Autodesk Fusion 360 part; units mm, degrees
sketch "スケッチ1" plane through (0, 0, 0) normal (0, 0, 1) x (1, 0, 0)
  line L0 (0, 0) -> (74, 0)
  line L1 (74, 0) -> (74, 46)
  line L2 (74, 46) -> (0, 46)
  line L3 (0, 46) -> (0, 0)
  dimension "d1" = 46
  dimension "d2" = 74
extrude "押し出し1" add sketch "スケッチ1" along normal blind 2
sketch "スケッチ2" plane through (0, 0, 2) normal (0, 0, 1) x (-1, 0, 0)
  line L0 (0, -46) -> (0, 0)
  line L1 (0, 0) -> (-74, 0)
  line L2 (-74, 0) -> (-74, -46)
  line L3 (-74, -46) -> (0, -46)
  line L4 (-27, -13) -> (-47, -13)
  line L5 (-47, -13) -> (-47, -15)
  line L6 (-47, -15) -> (-27, -15)
  line L7 (-27, -15) -> (-27, -13)
  dimension "d5" = 2
  dimension "d6" = 20
  dimension "d7" = 13
  dimension "d8" = 27
extrude "押し出し2" cut sketch "スケッチ2" against normal blind 2 contours L4 L5 L6 L7
sketch "スケッチ3" plane through (0, 0, 2) normal (0, 0, 1) x (-1, 0, 0)
  line L0 (-47, -13) -> (-27, -13)
  line L1 (-27, -13) -> (-27, -15)
  line L2 (-27, -15) -> (-47, -15)
  line L3 (-47, -15) -> (-47, -13)
  line L4 (0, -46) -> (0, 0)
  line L5 (0, 0) -> (-74, 0)
  line L6 (-74, 0) -> (-74, -46)
  line L7 (-74, -46) -> (0, -46)
  line L8 (-67, -46) -> (-58, -46)
  line L9 (-58, -46) -> (-58, -44)
  line L10 (-58, -44) -> (-67, -44)
  line L11 (-67, -44) -> (-67, -46)
  line L12 (-50, -46) -> (-41, -46)
  line L13 (-50, -44) -> (-50, -46)
  line L14 (-41, -44) -> (-50, -44)
  line L15 (-41, -46) -> (-41, -44)
  line L16 (-33, -46) -> (-24, -46)
  line L17 (-33, -44) -> (-33, -46)
  line L18 (-24, -44) -> (-33, -44)
  line L19 (-24, -46) -> (-24, -44)
  line L20 (-16, -46) -> (-7, -46)
  line L21 (-16, -44) -> (-16, -46)
  line L22 (-7, -44) -> (-16, -44)
  line L23 (-7, -46) -> (-7, -44)
  line L24 (-24, 0) -> (-33, 0)
  line L25 (-33, 0) -> (-33, -2)
  line L26 (-58, 0) -> (-67, 0)
  line L27 (-50, 0) -> (-50, -2)
  line L28 (-50, -2) -> (-41, -2)
  line L29 (-7, -2) -> (-7, 0)
  line L30 (-7, 0) -> (-16, 0)
  line L31 (-16, 0) -> (-16, -2)
  line L32 (-33, -2) -> (-24, -2)
  line L33 (-67, 0) -> (-67, -2)
  line L34 (-41, -2) -> (-41, 0)
  line L35 (-16, -2) -> (-7, -2)
  line L36 (-24, -2) -> (-24, 0)
  line L37 (-41, 0) -> (-50, 0)
  line L38 (-67, -2) -> (-58, -2)
  line L39 (-58, -2) -> (-58, 0)
  line L40 (0, -38) -> (-2, -38)
  line L41 (-2, -38) -> (-2, -32)
  line L42 (-2, -32) -> (0, -32)
  line L43 (0, -32) -> (0, -38)
  line L44 (-2, -20) -> (0, -20)
  line L45 (-2, -26) -> (-2, -20)
  line L46 (0, -26) -> (-2, -26)
  line L47 (0, -20) -> (0, -26)
  line L48 (-2, -8) -> (0, -8)
  line L49 (-2, -14) -> (-2, -8)
  line L50 (0, -14) -> (-2, -14)
  line L51 (0, -8) -> (0, -14)
  line L52 (-74, -20) -> (-72, -20)
  line L53 (-72, -8) -> (-72, -14)
  line L54 (-74, -8) -> (-72, -8)
  line L55 (-72, -14) -> (-74, -14)
  line L56 (-74, -38) -> (-74, -32)
  line L57 (-72, -32) -> (-72, -38)
  line L58 (-72, -26) -> (-74, -26)
  line L59 (-74, -32) -> (-72, -32)
  line L60 (-74, -14) -> (-74, -8)
  line L61 (-72, -20) -> (-72, -26)
  line L62 (-74, -26) -> (-74, -20)
  line L63 (-72, -38) -> (-74, -38)
  dimension "d11" = 9
  dimension "d12" = 2
  dimension "d13" = 7
  dimension "d16" = 17
  dimension "d17" = 0
  dimension "d20" = 0
  dimension "d21" = 44
  dimension "d22" = 6
  dimension "d23" = 2
  dimension "d24" = 8
  dimension "d27" = 0
  dimension "d28" = 12
  dimension "d31" = -72
  dimension "d32" = 0
extrude "押し出し3" cut sketch "スケッチ3" against normal blind 2 contours L4 L40 L41 L42 L43 | L7 L20 L21 L22 L23 | L4 L44 L45 L46 L47 | L7 L16 L17 L18 L19 | L4 L48 L49 L50 L51 | L7 L12 L13 L14 L15 | L7 L8 L9 L10 L11 | L5 L29 L30 L31 L35 | L5 L24 L25 L32 L36 | L6 L56 L57 L59 L63 | L5 L27 L28 L34 L37 | L6 L52 L58 L61 L62 | L5 L26 L33 L38 L39 | L6 L53 L54 L55 L60
The listing builds one solid part. Answer for the finished solid, in the listing's coordinates (mm). A direction names the side the tool comes from. Coordinates: 2 decimals unless noted, no trailing zeros. Write each loop counter-clockwise with the first axis right and the second up, starting at its lowest first coordinate (ties: lowest second). Pieces come first, ordered by that corner, then holes. Notation, with made-up numbers: M 59.25,57 L 109.25,57 A19 ccw 109.25,81 Z; hole C -14,30.25 d8. An arc over 180 degrees is marked long. Write each question's results on one line, items separated by ' | '.
Item 1: The part is cut by section A-A on x = 28. Determine the outline of the cut face in (y, z).
Answer below:
outline: M 2,0 L 13,0 L 13,2 L 2,2 Z; M 15,0 L 44,0 L 44,2 L 15,2 Z
Item 2: For a pull along Y with two mould halves and no side action, classify faces 1 (the face through (62, 44, 1)), 2 (the face through (73, 14, 1)), 3 (the face through (74, 17, 1)), 4 (the face through (72, 35, 1)) as released by +Y, released by -Y, zero draft, split by the parting line, or undercut.
Answer below:
face 1: released by +Y | face 2: undercut | face 3: zero draft | face 4: undercut
Item 3: Consider probe 1 along Y at (x, z) = (36.5, 0.45); probe 2 along X at (y, z) = (13.5, 1); probe 3 along Y at (x, z) = (61.5, 0.35). Determine where each line is inside the solid, lowest interval first. Write a range as [from, to].
Answer below:
probe 1: [0, 13], [15, 46] | probe 2: [2, 27], [47, 72] | probe 3: [2, 44]
Item 4: Which of the six approach directions +Z, -Z, +X, -X, +Y, -Y give full straight-line access (tool end or side, diameter ignored) to faces 5 (the face through (72, 11, 1)), 6 (the face through (1, 32, 1)), 7 (the face through (50, 1, 1))?
Answer below:
face 5: +Z, -Z, +X | face 6: +Z, -Z, -X | face 7: +Z, -Z, -Y
Item 5: Given P1, Ø1, axis at y = 45, z = 1.5, coming from the -X side; P2, Ø0.6, axis at x = 27, z = 1, coming from the -Y side; P3, Ø0.6, axis at y = 12.5, z = 1, coming from the +X side, each flat-ended and moving along its own axis, determine where each tip first touches the part or whether it passes through.
Answer below:
P1: x = 0 | P2: y = 2 | P3: x = 72
Item 6: The part is cut by section C-C on x = 64. Determine the outline of the cut face in (y, z), and give its area (3 significant figures).
Answer below:
outline: M 2,0 L 44,0 L 44,2 L 2,2 Z | area: 84.0 mm2
Item 7: The part is cut by section B-B on y = 25. Determine the outline of the cut face in (x, z), and give its area (3 significant figures).
Answer below:
outline: M 2,0 L 72,0 L 72,2 L 2,2 Z | area: 140 mm2
